CAD build for the part. Positions are in the model's coordinates, mm. A direction names the side the tool comes from. Coordinates: 2 decimals unless noted, no trailing zeros. Loops run counter-clockwise (first coordinate to the right, second up) from the corner with the lowest first, then second, coordinate; pieces in that order, holes last. Notation, with made-up numbers: (2.25, -20) -> (7.25, -20) arc R7 ccw to (7.25, -9) -> close; hole circle Ø8 at (38, 52). An arc over 180 degrees is marked (long way). Return JSON: item names as keys, results as strings. Group by question number.
(1) Tool access for faces 4 (the face through (-15, 10, -30)), 5 (the face through (-30, 10, -99)): list every direction of +Z, -Z, +X, -X, +Y, -Y with a clear straight run to the whole face (end or side of a thin tool).
(2) Saw through at B-B on x = -15. Write the cut outline in (y, z).
(3) Saw through at A-A on z = -33. Write the cut outline in (x, y).
(4) Probe L1, parallel to Z at x = -15, y = 18; L2, parallel to Z at x = -19, y = 15.25. List the from-to ranges inside material, lowest first.
(5) Mould opens along Z. For faces 1 (the face through (-16.08, 15.07, -25.12)), 2 (the face through (-15, 20, -99)), 3 (the face through (-15, 10, -200)) say: pulls with the +Z half, pulls with the -Z half, needs draft (parallel to the pull), parting line crosses it, or undercut.
Autodesk Inventor part; units mm, degrees
ref_plane "YZ Plane" through (0, 0, 0) normal (1, 0, 0) x (0, 1, 0)
ref_plane "XZ Plane" through (0, 0, 0) normal (0, 1, 0) x (-1, 0, 0)
ref_plane "XY Plane" through (0, 0, 0) normal (0, 0, 1) x (1, 0, 0)
sketch "Esboço1" plane through (0, 0, 0) normal (0, 1, 0) x (-1, 0, 0)
  line L0 (0, 0) -> (30, 0)
  line L1 (30, 0) -> (30, -200)
  line L2 (30, -200) -> (0, -200)
  line L3 (0, -200) -> (0, 0)
  dimension "d0" = 30
  dimension "d1" = 200
extrude "Extrusão1" add sketch "Esboço1" along normal blind 20
sketch "Esboço2" plane through (0, 20, 0) normal (0, 1, 0) x (1, 0, 0)
  line L0 (-30, 0) -> (0, 0)
  line L1 (-15, 0) -> (-15, 30)
  circle A0 centre (-15, 30) radius 5
  dimension "d4" = 30
  dimension "d5" = 10
extrude "Extrusão2" cut sketch "Esboço2" against normal blind 10
properties part number "Superior"
Geometry results:
{
 "1": {"face 4": "+Y", "face 5": "+Z, -Z, -X, +Y, -Y"},
 "2": {"outline": "(0, -200) -> (20, -200) -> (20, -35) -> (10, -35) -> (10, -25) -> (20, -25) -> (20, 0) -> (0, 0) -> close"},
 "3": {"outline": "(-30, 0) -> (0, 0) -> (0, 20) -> (-11, 20) -> (-11, 10) -> (-19, 10) -> (-19, 20) -> (-30, 20) -> close"},
 "4": {"L1": "-200 to -35, -25 to 0", "L2": "-200 to -33, -27 to 0"},
 "5": {"face 1": "undercut", "face 2": "needs draft", "face 3": "pulls with the -Z half"}
}
